from build123d import *

# Parameters (mm, degrees)
SKETCH_1_W         = 25
SKETCH_1_H         = 8
EXTRUDE_1_DEPTH    = 8
CHAMFER_1_SIZE     = 0.5
HOLE_WIZARD_M4_1_D = 3.3
HOLE_WIZARD_M4_2_D = 3.3


with BuildPart() as part:
    # 草图1 → 凸台-拉伸1 (new body)
    with BuildSketch(Plane.XY):
        Rectangle(SKETCH_1_W, SKETCH_1_H)
    extrude(amount=EXTRUDE_1_DEPTH)

    # 倒角1
    chamfer_1_edges = [part.edges().sort_by_distance(p)[0] for p in [
        (-12.5, 0, 8),
        (0, -4, 8),
        (12.5, 0, 8),
        (0, -4, 0),
        (-12.5, 0, 0),
        (0, 4, 0),
        (12.5, 0, 0),
        (12.5, -4, 4),
        (-12.5, -4, 4),
        (-12.5, 4, 4),
        (12.5, 4, 4),
        (0, 4, 8),
    ]]
    chamfer(chamfer_1_edges, length=CHAMFER_1_SIZE)

    # M4 螺纹孔1 (through all)
    with Locations(Plane(origin=(0, -4, 4), x_dir=(0, 0, -1), z_dir=(0, -1, 0))):
        with Locations((0, 0)):
            Hole(HOLE_WIZARD_M4_1_D / 2)

    # M4 螺纹孔2 (through all)
    with Locations(Plane(origin=(-7.5, 0, 8), x_dir=(1, 0, 0), z_dir=(0, 0, 1))):
        with Locations((0, 0), (15, 0)):
            Hole(HOLE_WIZARD_M4_2_D / 2)


solid = part.part
Model file for the job. Use its own axes, mm. Give positions to 0.01 mm unless a question says otherwise; leave off trailing zeros. Loops run counter-clockwise (first coordinate to the right, second up) from the corner with the lowest first, then second, coordinate; pieces in that order, holes last. Notation, with made-up numbers: (67, 47.5) -> (84, 47.5) arc R21 cw to (84, 57.5) -> close; hole circle Ø5 at (72, 24). An arc over 180 degrees is marked (long way). Use a Markdown table: item, result. Add a question column.
(1) Slice it at D-D on z = 1.5. List the corners of the cut face in (x, y).
(2) Drop a flat-ended pin along its axis: pin 1 Ø2.5 at (x, z) = (0, 4) entering from -Y. Give the stop position or say it passes through.
(3) Slice it at A-A on z = 4. List the corners of the cut face in (x, y).
(4) Slice it at C-C on y = -2. List the corners of the cut face in (x, z), and give its area (3 significant figures).
(5) Slice it at B-B on x = 0. List the corners of the cut face in (y, z), and give its area (3 significant figures).
(6) Wall check: line 1 along X through (y, z) = (1, 6); line 2 along X through (y, z) = (1.75, 4); line 3 along X through (y, z) = (-1.25, 4). Give the ranges that are in metal, low to high.
(7) Mould opens along Y. For faces 1 (the flat face through (0, 4, 2)), 2 (the cylindrical face through (-5.85, 0.07, 3.94)), 3 (the cylindrical face through (0.07, 0.06, 2.35)) say: +Y half, -Y half, draft (parallel to the pull), parting line (faces both ways), or undercut.
Filled sheet:
| question | item | result |
|---|---|---|
| 1 | outline | (-12.5, -3.5) -> (-12, -4) -> (12, -4) -> (12.5, -3.5) -> (12.5, 3.5) -> (12, 4) -> (-12, 4) -> (-12.5, 3.5) -> close; hole circle Ø3.3 at (-7.5, 0); hole circle Ø3.3 at (7.5, 0) |
| 2 | pin 1 | through |
| 3 | outline | (-12.5, -3.5) -> (-12, -4) -> (-1.65, -4) -> (-1.65, 4) -> (-12, 4) -> (-12.5, 3.5) -> close; (1.65, -4) -> (12, -4) -> (12.5, -3.5) -> (12.5, 3.5) -> (12, 4) -> (1.65, 4) -> close; hole circle Ø3.3 at (-7.5, 0); hole circle Ø3.3 at (7.5, 0) |
| 4 | outline | (-12.5, 0.5) -> (-12, 0) -> (12, 0) -> (12.5, 0.5) -> (12.5, 7.5) -> (12, 8) -> (-12, 8) -> (-12.5, 7.5) -> close; hole circle Ø3.3 at (0, 4) |
| 4 | area | 191 mm2 |
| 5 | outline | (-4, 0.5) -> (-3.5, 0) -> (3.5, 0) -> (4, 0.5) -> (4, 2.35) -> (-4, 2.35) -> close; (-4, 5.65) -> (4, 5.65) -> (4, 7.5) -> (3.5, 8) -> (-3.5, 8) -> (-4, 7.5) -> close |
| 5 | area | 37.1 mm2 |
| 6 | line 1 | -12.5 to -8.81, -6.19 to 6.19, 8.81 to 12.5 |
| 6 | line 2 | -12.5 to -1.65, 1.65 to 12.5 |
| 6 | line 3 | -12.5 to -8.58, -6.42 to -1.65, 1.65 to 6.42, 8.58 to 12.5 |
| 7 | face 1 | +Y half |
| 7 | face 2 | undercut |
| 7 | face 3 | draft |
